```python
from build123d import *

# Parameters (mm, degrees)
CYLINDER007_R     = 1.55
CYLINDER007_DEPTH = 10
CYLINDER006_R     = 1.55
CYLINDER006_DEPTH = 10
BOX003_W          = 10
BOX003_H          = 50
BOX003_DEPTH      = 2


with BuildPart() as cylinder007:
    # Cylinder007 → Cylinder007 (new body)
    with BuildSketch(Plane(origin=(-5, 38, 14), x_dir=(1, 0, 0), z_dir=(0, 0, 1))):
        Circle(CYLINDER007_R)
    extrude(amount=CYLINDER007_DEPTH)


with BuildPart() as cylinder006:
    # Cylinder006 → Cylinder006 (new body)
    with BuildSketch(Plane(origin=(-5, 12, 14), x_dir=(1, 0, 0), z_dir=(0, 0, 1))):
        Circle(CYLINDER006_R)
    extrude(amount=CYLINDER006_DEPTH)


with BuildPart() as lip018:
    # Box003 → Box003 (new body)
    with BuildSketch(Plane(origin=(-10, 0, 18), x_dir=(1, 0, 0), z_dir=(0, 0, 1))):
        with Locations((5, 25)):
            Rectangle(BOX003_W, BOX003_H)
    extrude(amount=BOX003_DEPTH)

    # Cut006: cut Cylinder006
    add(cylinder006.part, mode=Mode.SUBTRACT)

    # Cut007: cut Cylinder007
    add(cylinder007.part, mode=Mode.SUBTRACT)


solid = lip018.part
```
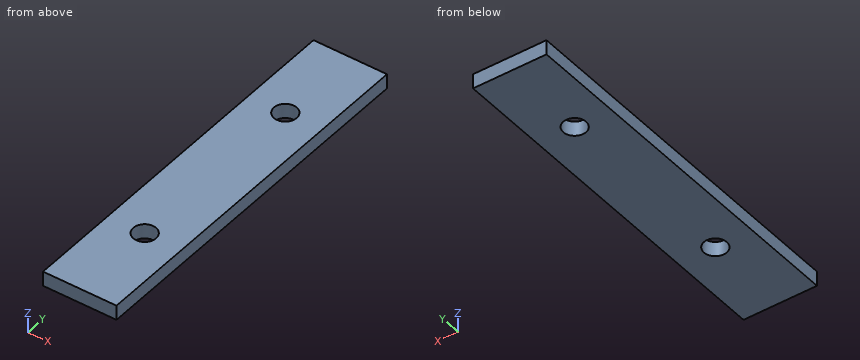
Geometry: final body of the model. Coordinates: model frame, mm. Round coordinates to 2 decimals unless told otherwise and drop trailing zeros. Order: outer loops, then holes, each group sorted by start corner. A loop starts at its lowest first (then second) coordinate and runs counter-clockwise, first axis right, second up. Notation, with made-up numbers: (-35, 29.25) - (2, 29.25) arc R25 cw to (2, 64.25) - close; hole circle Ø2 at (87.5, -26.75). An arc over 180 degrees is marked (long way). Write item = value, one per line. Start each with the question number.
Q1. Cut plane A-A on x = -5. Return the cut outline in (y, z), and give its area (3 significant figures).
Q2. Ray query, line 1 (Y direction, x = -5, z = 19); line 2 (X direction, y = 12, z = 18.8). Return the intervals inside material, ascending. Write a range as from..to.
Q3. Pin query (flat end, axial travel): pin 1 (1 mm diameter, centred on x = -3, z = 18.5, fed in from -Y); pin 2 (3 mm diameter, centred on x = -5, y = 12, fed in from +Z). Return the tip coordinate at first contact, or that it passes through.
Q4. Cut plane B-B on y = 38. Return the cut outline in (x, z).
Q5. Cut plane C-C on z = 19.5. Return the cut outline in (x, y), and give its area (3 significant figures).
Outcome:
q1.outline = (0, 18) - (10.45, 18) - (10.45, 20) - (0, 20) - close; (13.55, 18) - (36.45, 18) - (36.45, 20) - (13.55, 20) - close; (39.55, 18) - (50, 18) - (50, 20) - (39.55, 20) - close
q1.area = 87.6 mm^2
q2.line_1 = 0..10.45, 13.55..36.45, 39.55..50
q2.line_2 = -10..-6.55, -3.45..0
q3.pin_1 = 0
q3.pin_2 = through
q4.outline = (-10, 18) - (-6.55, 18) - (-6.55, 20) - (-10, 20) - close; (-3.45, 18) - (0, 18) - (0, 20) - (-3.45, 20) - close
q5.outline = (-10, 0) - (0, 0) - (0, 50) - (-10, 50) - close; hole circle Ø3.1 at (-5, 12); hole circle Ø3.1 at (-5, 38)
q5.area = 485 mm^2
